Drawing for the job (mm, zero at the part's lowest x, y, z). A direction names the side the tool comes from. Give positions to 0.01 mm unless a question says otherwise; leave off trailing zeros. Use a Markdown table: item, result. Add a question column.
(1) Flat gauge pins, fed straight in: pin 1 (15 mm diameter, centred on x = 80.5, z = 37.5, fed in from +Y); pin 2 (24 mm diameter, centred on x = 151, z = 15, fed in from -Y); pin 3 (4 mm diameter, centred on y = 2, z = 33.5, fed in from -X). Where does each tip first touch, or does it go through?
(2) Mould opens along X. For the marked faces 1 and 2 say: +X half, -X half, draft (parallel to the pull), parting line (faces both ways), or undercut.
(3) Which spindle directions (+Z, -Z, +X, -X, +Y, -Y) get a long thin tool onto all of the face, cutting with end or side? Do the marked faces 3 and 4. Say none if no direction does.
(4) Slice it at A-A (z = 12.7). Count the separate pieces of the cut face and the enclosed holes in it, then the cut area to 3 significant figures.
(5) Wall check: line 1 (X direction, y = 11.25, z = 38.1); line 2 (X direction, y = 3, z = 38) (1 decimal); line 3 (X direction, y = 10, z = 38.5). Give the ranges that are in metal, low to high.
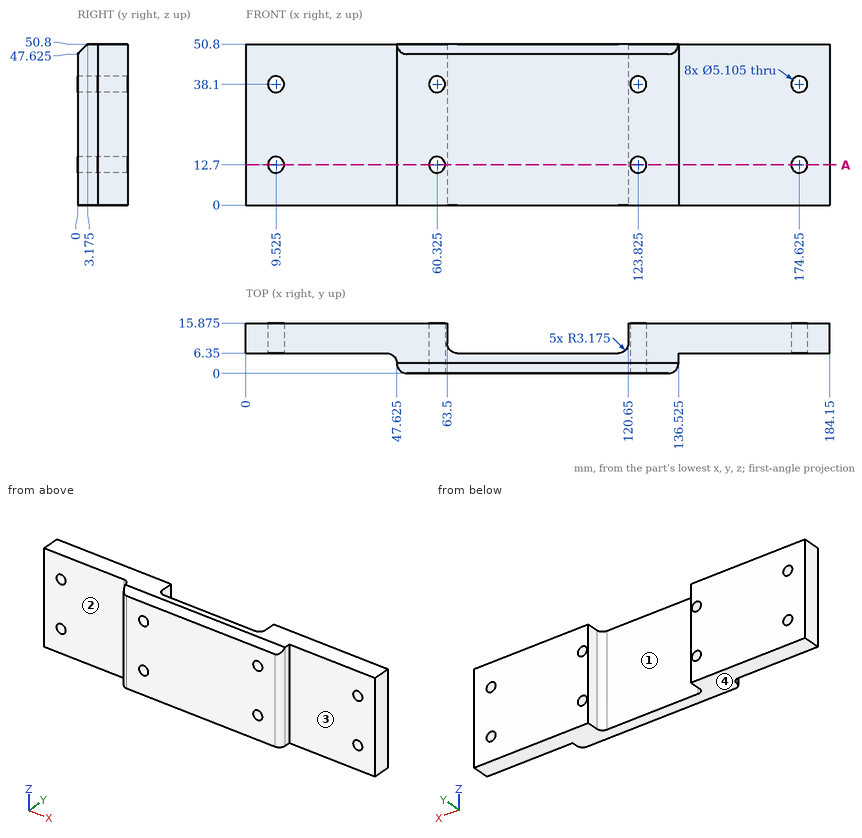
Solution:
| question | item | result |
|---|---|---|
| 1 | pin 1 | y = 6.35 |
| 1 | pin 2 | y = 6.35 |
| 1 | pin 3 | x = 47.52 |
| 2 | face 1 | undercut |
| 2 | face 2 | draft |
| 3 | face 3 | +Z, -Z, +X, -Y |
| 3 | face 4 | -Z, +X, -X, +Y, -Y |
| 4 | separate pieces | 5 |
| 4 | enclosed holes | 0 |
| 4 | area | 1,520 mm2 |
| 5 | line 1 | 0 to 6.97, 12.08 to 57.77, 62.88 to 63.5, 120.65 to 121.27, 126.38 to 172.07, 177.18 to 184.15 |
| 5 | line 2 | 47.6 to 57.8, 62.9 to 121.3, 126.4 to 136.5 |
| 5 | line 3 | 0 to 7, 12.05 to 57.8, 62.85 to 63.5, 120.65 to 121.3, 126.35 to 172.1, 177.15 to 184.15 |
